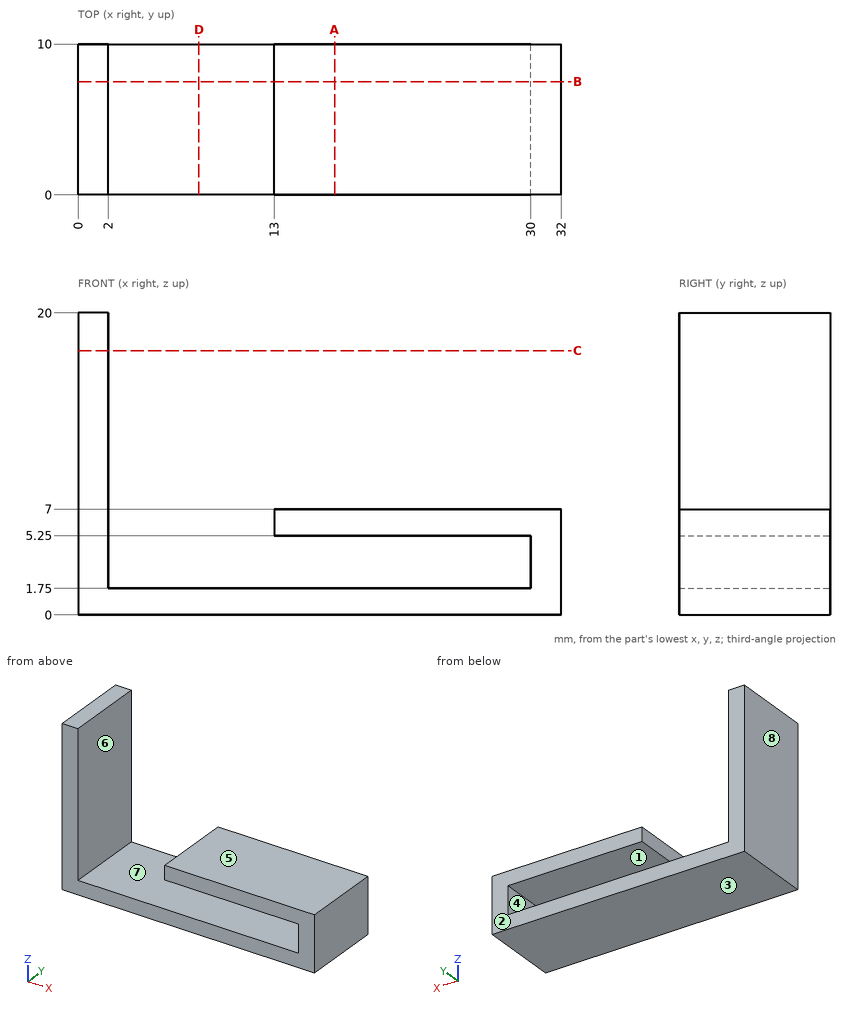
Verification items for this drawing (mm, ordinates from the low corner). A direction names the side the tool comes from. Give positions to 0.01 mm unless a question says otherwise; leave off trailing zeros. Write each loop counter-clockwise with the first axis right and the second up, starting at its lowest first coordinate (ties: lowest second). Pieces come first, ordered by that corner, then holes.
1) Set-up check for the marked faces 5, 6, 7 and 8: record each of +Z, -Z, +X, -X, +Y, -Y from which the full face is reachable in a straight line by a thin tool's end or side.
Values follow:
face 5: +Z, +X, +Y, -Y
face 6: +Z, +Y, -Y
face 7: +Y, -Y
face 8: +Z, -Z, -X, +Y, -Y
2) Go/stop test with flat-tipped pins: pin 1 Ø3 at (x, y) = (21.5, 2.5) entering from +Z; pin 2 Ø1.5 at (y, z) = (5, 15.5) entering from +X. Record where each tip stops, or that it passes through.
Values follow:
pin 1: stops at z = 7
pin 2: stops at x = 2
3) Thickness scan on line 1 (X direction, y = 9.75, z = 5.5); line 2 (Z direction, x = 19.5, y = 5.25); line 3 (X direction, y = 4, z = 2). Record the ranges inside material, lowest first.
Values follow:
line 1: x = 0 to 2, 13 to 32
line 2: z = 0 to 1.75, 5.25 to 7
line 3: x = 0 to 2, 30 to 32
4) Cross-section at A-A (x = 17). Record the boundary of the cut face in (y, z), plus the area to 3 significant figures.
Values follow:
outline: (0, 0) - (10, 0) - (10, 1.75) - (0, 1.75) - close; (0, 5.25) - (10, 5.25) - (10, 7) - (0, 7) - close
area: 35.0 mm2
5) Cross-section at C-C (z = 17.5). Record the boundary of the cut face in (x, y).
Values follow:
outline: (0, 0) - (2, 0) - (2, 10) - (0, 10) - close
6) Cross-section at D-D (x = 8). Record the boundary of the cut face in (y, z), plus the area to 3 significant figures.
Values follow:
outline: (0, 0) - (10, 0) - (10, 1.75) - (0, 1.75) - close
area: 17.5 mm2
7) Release check for a two-part mould opening along Z. For the marked faces 1, 2, 3 and 4 record: released by +Z, released by -Z, zero draft, split by the parting line, or undercut.
Values follow:
face 1: undercut
face 2: zero draft
face 3: released by -Z
face 4: undercut
8) Cross-section at B-B (y = 7.5). Record the boundary of the cut face in (x, z), plus the area to 3 significant figures.
Values follow:
outline: (0, 0) - (32, 0) - (32, 7) - (13, 7) - (13, 5.25) - (30, 5.25) - (30, 1.75) - (2, 1.75) - (2, 20) - (0, 20) - close
area: 133 mm2
